Part print with two shaded views. Sizes in mm from the minimum x, y, z corner. Round coordinates to 2 decimals unless told otherwise and drop trailing zeros. Loops run counter-clockwise (first coordinate to the right, second up) from the corner with the lowest first, then second, coordinate; pieces in that order, holes last. Notation, with made-up numbers: (60.5, 72.25) -> (107.5, 72.25) arc R33 cw to (107.5, 109.25) -> close; hole circle Ø3 at (66.25, 75). An arc over 180 degrees is marked (long way). Use a Markdown table: item, result. Add a question column.
Item 1: Cut at C-C, the plane x = 360. List the corners of the cut face in (y, z), plus the area to 3 significant figures.
Item 2: Probe line 1 (Z direction, x = 226, y = 124.5); line 2 (Y direction, x = 56.5, z = 151.5); line 3 (Y direction, x = 346, z = 153). List the from-to ranges inside material, lowest first. Write a range as [from, to].
Item 3: Cut at A-A, the plane z = 125. List the corners of the cut face in (x, y), plus the area to 3 significant figures.
Item 4: Two-plate mould, pull along Z, no slides. Class the marked faces 1, 2, 3 and 4: pulls with the +Z half, pulls with the -Z half, needs draft (parallel to the pull), parting line crosses it, or undercut.
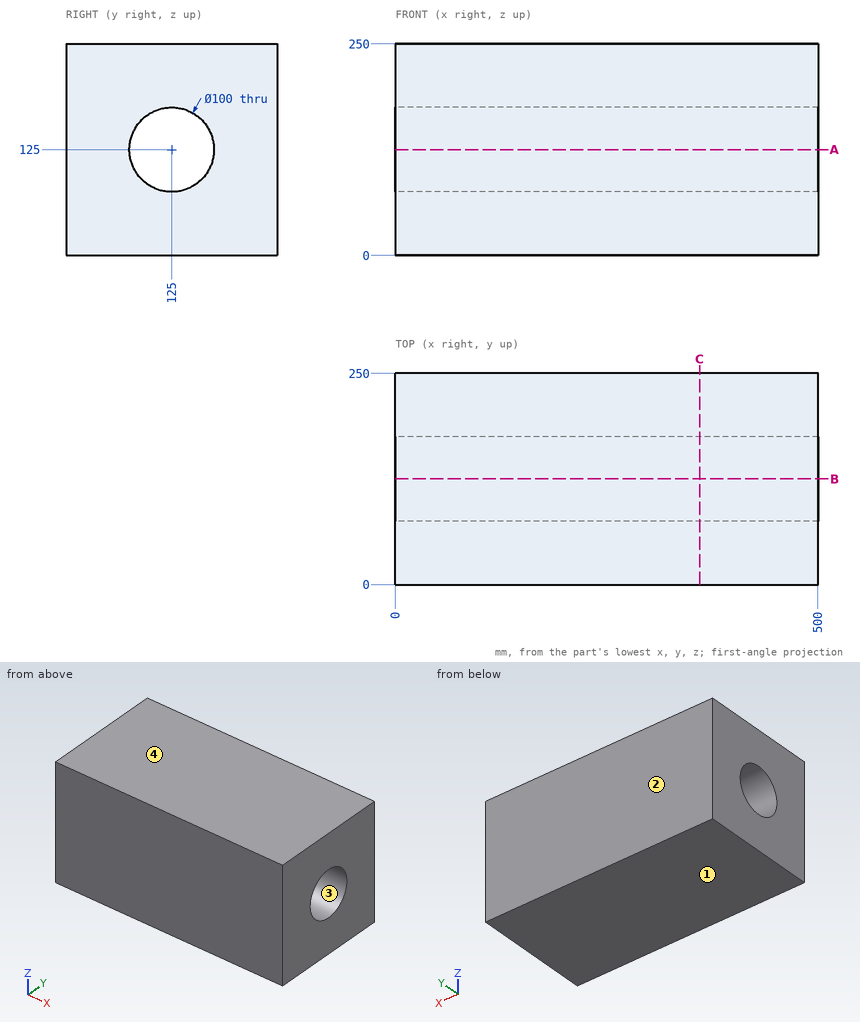
A:
| question | item | result |
|---|---|---|
| 1 | outline | (0, 0) -> (250, 0) -> (250, 250) -> (0, 250) -> close; hole circle Ø100 at (125, 125) |
| 1 | area | 54,600 mm^2 |
| 2 | line 1 | z = [0, 75], [175, 250] |
| 2 | line 2 | y = [0, 82.6], [167.4, 250] |
| 2 | line 3 | y = [0, 83.58], [166.42, 250] |
| 3 | outline | (0, 0) -> (500, 0) -> (500, 75) -> (0, 75) -> close; (0, 175) -> (500, 175) -> (500, 250) -> (0, 250) -> close |
| 3 | area | 75,000 mm^2 |
| 4 | face 1 | pulls with the -Z half |
| 4 | face 2 | needs draft |
| 4 | face 3 | undercut |
| 4 | face 4 | pulls with the +Z half |
